Design review of the part built by this model. Coordinates are the model's own, in mm. A direction names the side the tool comes from. Round coordinates to 2 decimals unless told otherwise and drop trailing zeros. Order: outer loops, then holes, each group sorted by start corner. A loop starts at its lowest first (then second) coordinate and runs counter-clockwise, first axis right, second up. Notation, with made-up numbers: (-3, -11) - (16, -11) arc R27 cw to (16, 7) - close; hole circle Ø10 at (-28.75, -13). An arc over 180 degrees is marked (long way). Use CSV: the item, a comma, the result in double quotes.
from build123d import *

# Parameters (mm, degrees)
SM_BASE_FLANGE_1_DEPTH = 8
CUT_EXTRUDE_1_DEPTH    = 10


# Sheet-metal steps are written as plain solids
with BuildPart() as part:
    # Sketch 1 → Базовая кромка1 (new body)
    with BuildSketch(Plane.XY):
        Polygon((0, 0), (0, 120), (110, 120), (110, 68.738635424), (60, 0), align=None)
    extrude(amount=-SM_BASE_FLANGE_1_DEPTH)

    # Эскиз6 → Вырез-Вытянуть1 (cut)
    with BuildSketch(Plane.XY):
        with BuildLine():
            Line((66.474866664, 63.30146998), (75.298396076, 75.431817408))
            ThreePointArc((75.298396076, 75.431817408), (85.076871934, 76.974999149), (86.620053675, 67.196523291))
            Line((86.620053675, 67.196523291), (77.796524263, 55.066175863))
            ThreePointArc((77.796524263, 55.066175863), (68.018048405, 53.522994122), (66.474866664, 63.30146998))
        make_face()
        with BuildLine():
            Line((51.768984311, 43.084224267), (42.945454899, 30.95387684))
            ThreePointArc((42.945454899, 30.95387684), (44.48863664, 21.175400981), (54.267112498, 22.718582722))
            Line((54.267112498, 22.718582722), (63.09064191, 34.84893015))
            ThreePointArc((63.09064191, 34.84893015), (61.547460169, 44.627406008), (51.768984311, 43.084224267))
        make_face()
    extrude(amount=-CUT_EXTRUDE_1_DEPTH, mode=Mode.SUBTRACT)


solid = part.part
1) We need section B-B (z = -3.25). Give the boundary of the cut face in (x, y), then the cut area to 3 significant figures.
Data:
outline,"(0, 0) - (60, 0) - (110, 68.74) - (110, 120) - (0, 120) - close; hole (42.95, 30.95) arc R7 ccw to (54.27, 22.72) - (63.09, 34.85) arc R7 ccw to (51.77, 43.08) - close; hole (66.47, 63.3) arc R7 ccw to (77.8, 55.07) - (86.62, 67.2) arc R7 ccw to (75.3, 75.43) - close"
area,"10,800 mm2"
2) The part is to be moulded in two halves that separate along X. For faces 3 (the face through (47.419, 37.104, -3.944)), 4 (the face through (54, 120, -4)), 5 (the face through (110, 95, -4)), say which applies: +X half, -X half, draft (parallel to the pull), parting line (faces both ways), or undercut.
Data:
face 3,"undercut"
face 4,"draft"
face 5,"+X half"
3) For faces 1 (the face through (0, 59, -4)), 2 (the face through (58.62, 28.7, -3.94)), list the 3-axis set-ups (+Z, -Z, +X, -X, +Y, -Y) from which the entire face can be reached by the end or side of a thin tool; tool diameter is ignored.
Data:
face 1,"+Z, -Z, -X, +Y, -Y"
face 2,"+Z, -Z"
4) Insertion check: pin 1 Ø3 at (x, z) = (85, -2) entering from -Y; pin 2 Ø1 at (y, z) = (32.5, -1.5) entering from +X. Each pin has a flat end and moves straight along its axis. Give the tip position at first contact, or say it passes through.
Data:
pin 1,"stops at y = 32.31"
pin 2,"stops at x = 84"
5) We need section C-C (y = 39). Give the boundary of the cut face in (x, z).
Data:
outline,"(0, -8) - (48.8, -8) - (48.8, 0) - (0, 0) - close; (64.43, -8) - (88.37, -8) - (88.37, 0) - (64.43, 0) - close"
6) To check wall thickness, follow L1, parallel to Y at x = 42.5, z = -3.5; L2, parallel to X at y = 53, z = -2.25; L3, parallel to X at y = 72.5, z = -1.25. State the ranges of each line that lie inside material, in increasing order. Write a range as from..to.
Data:
L1,"y = 0..23.41, 30.26..120"
L2,"x = 0..68.86, 75.42..98.55"
L3,"x = 0..73.17, 87.86..110"
7) We need section A-A (x = 46). Give the boundary of the cut face in (y, z), then the cut area to 3 significant figures.
Data:
outline,"(0, -8) - (20.34, -8) - (20.34, 0) - (0, 0) - close; (35.15, -8) - (120, -8) - (120, 0) - (35.15, 0) - close"
area,"841 mm2"
